Verification items for the finished model (mm, model axes). Face numbers are marked on the shaded views. A direction names the side the tool comes from. Round coordinates to 2 decimals unless told otherwise and drop trailing zeros. Write each loop counter-clockwise with the first axis right and the second up, starting at its lowest first coordinate (ties: lowest second). Pieces come first, ordered by that corner, then holes. Notation, with made-up numbers: M 76.5,68.5 L 116.5,68.5 A33 ccw 116.5,103.5 Z; hole C 39,81 d2. An arc over 180 degrees is marked long. Answer in a Markdown table with one row per item. Add a question column.
1. Go/stop test with flat-tipped pins: pin 1 Ø8 at (x, z) = (-8.5, 4) entering from +Y; pin 2 Ø8 at (y, z) = (13, 12.5) entering from +X; pin 3 Ø5 at (x, z) = (0, -5) entering from -Y; pin 4 Ø5 at (y, z) = (20.5, 10.5) entering from -X. Record where each tip stops, or that it passes through.
2. Material ranges on probe 1 along X at (y, z) = (2.75, -5); probe 2 along X at (y, z) = (6.5, -4); probe 3 along Z at (x, y) = (18.4, 2.75), recorded low to high.
3. Set-up check for the marked faces 5, 6, 7, 8 and 9: record each of +Z, -Z, +X, -X, +Y, -Y from which the full face is reachable in a straight line by a thin tool's end or side.
4. Sectioned sample at A-A on x = 0. Count the separate pieces of the cut face and the enclosed holes in it, plus the area to 3 significant figures.
5. Draft check along Z on the marked faces 1, 2, 3 and 4. Enter one of: pulls with the +Z half, pulls with the -Z half, needs draft (parallel to the pull), parting line crosses it, or undercut.
6. Sectioned sample at B-B on x = -18.4. Record the cut outline in (y, z), plus the area to 3 significant figures.
7. Sectioned sample at D-D on z = -4.5. Record the cut outline in (x, y).
8. Sectioned sample at C-C on y = 20.5. Record the cut outline in (x, z).
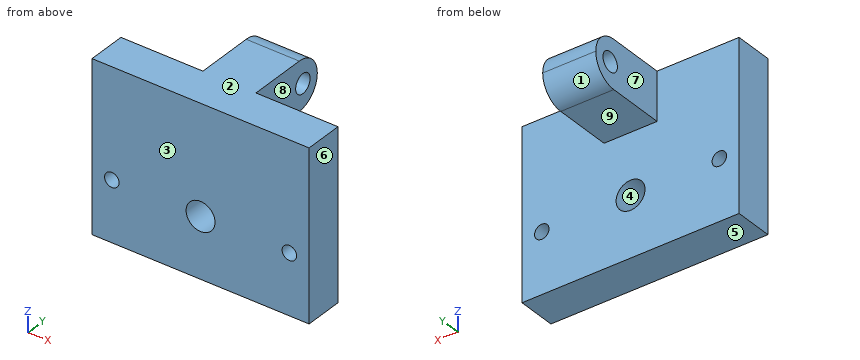
```python
from build123d import *

# Parameters (mm, degrees)
SKETCH2_W           = 45
SKETCH2_H           = 35
SKETCH2_R           = 3
SKETCH2_R_2         = 1.5
BOSS_EXTRUDE1_DEPTH = 5
SKETCH4_R           = 1.5
SKETCH4_R_2         = 3
SKETCH4_W           = 11
SKETCH4_H           = 10
BOSS_EXTRUDE2_DEPTH = 3
SKETCH4_3_W         = 11
SKETCH4_3_H         = 10
BOSS_EXTRUDE3_DEPTH = 20
SKETCH5_R           = 2
CUT_EXTRUDE1_DEPTH  = 20
FILLET1_R           = 5


with BuildPart() as part:
    # Sketch2 → Boss-Extrude1 (new body)
    with BuildSketch(Plane(origin=(0, 0, 0), x_dir=(1, 0, 0), z_dir=(0, 1, 0))):
        Rectangle(SKETCH2_W, SKETCH2_H)
        with Locations(Location((0, 5, 0), (0, 0, 270))):
            Circle(SKETCH2_R, mode=Mode.SUBTRACT)
        with Locations(Location((-18.4, 5, 0), (0, 0, 270))):
            Circle(SKETCH2_R_2, mode=Mode.SUBTRACT)
        with Locations(Location((18.4, 5, 0), (0, 0, 90))):
            Circle(SKETCH2_R_2, mode=Mode.SUBTRACT)
    extrude(amount=BOSS_EXTRUDE1_DEPTH)

    # Sketch4 → Boss-Extrude2 (add)
    # profile 1 of 3: a face of its own
    with BuildSketch(Plane(origin=(0, 5, 0), x_dir=(1, 0, 0), z_dir=(0, 1, 0))):
        Polygon((5.5, -17.5), (15, -17.5), (22.5, -17.5), (22.5, 17.5), (-22.5, 17.5), (-22.5, -17.5), (-15, -17.5), (-5.5, -17.5), (-5.5, -7.5), (5.5, -7.5), align=None)
        with Locations(Location((-18.4, 5, 0), (0, 0, 270))):
            Circle(SKETCH4_R, mode=Mode.SUBTRACT)
        with Locations(Location((0, 5, 0), (0, 0, 270))):
            Circle(SKETCH4_R_2, mode=Mode.SUBTRACT)
        with Locations(Location((18.4, 5, 0), (0, 0, 90))):
            Circle(SKETCH4_R, mode=Mode.SUBTRACT)
    # profile 2 of 3: a face of its own
    with BuildSketch(Plane(origin=(0, 5, 0), x_dir=(1, 0, 0), z_dir=(0, 1, 0))):
        Polygon((5.5, -17.5), (15, -17.5), (22.5, -17.5), (22.5, 17.5), (-22.5, 17.5), (-22.5, -17.5), (-15, -17.5), (-5.5, -17.5), (-5.5, -7.5), (5.5, -7.5), align=None)
        with Locations(Location((-18.4, 5, 0), (0, 0, 270))):
            Circle(SKETCH4_R, mode=Mode.SUBTRACT)
        with Locations(Location((0, 5, 0), (0, 0, 270))):
            Circle(SKETCH4_R_2, mode=Mode.SUBTRACT)
        with Locations(Location((18.4, 5, 0), (0, 0, 90))):
            Circle(SKETCH4_R, mode=Mode.SUBTRACT)
    # profile 3 of 3: a face of its own
    with BuildSketch(Plane(origin=(0, 5, 0), x_dir=(1, 0, 0), z_dir=(0, 1, 0))):
        with Locations((0, -12.5)):
            Rectangle(SKETCH4_W, SKETCH4_H)
    extrude(amount=BOSS_EXTRUDE2_DEPTH)

    # Sketch4<3> → Boss-Extrude3 (add)
    with BuildSketch(Plane(origin=(0, 5, 0), x_dir=(1, 0, 0), z_dir=(0, 1, 0))):
        with Locations((0, -12.5)):
            Rectangle(SKETCH4_3_W, SKETCH4_3_H)
    extrude(amount=BOSS_EXTRUDE3_DEPTH)

    # Sketch5 → Cut-Extrude1 (cut)
    with BuildSketch(Plane(origin=(5.5, 0, 0), x_dir=(0, 0, -1), z_dir=(1, 0, 0))):
        with Locations((-12.5, 21)):
            Circle(SKETCH5_R)
    extrude(amount=-CUT_EXTRUDE1_DEPTH, mode=Mode.SUBTRACT)

    # Fillet1
    fillet1_edges = [part.edges().sort_by_distance(p)[0] for p in [
        (0, 25, 7.5),
        (0, 25, 17.5),
    ]]
    fillet(fillet1_edges, radius=FILLET1_R - 0.0001)  # a hair under: the kernel refuses the full size


solid = part.part
```
Geometry check:
| question | item | result |
|---|---|---|
| 1 | pin 1 | stops at y = 8 |
| 1 | pin 2 | stops at x = 5.5 |
| 1 | pin 3 | passes through |
| 1 | pin 4 | stops at x = -5.5 |
| 2 | probe 1 | x = -22.5 to -19.9, -16.9 to -3, 3 to 16.9, 19.9 to 22.5 |
| 2 | probe 2 | x = -22.5 to -19.52, -17.28 to -2.83, 2.83 to 17.28, 19.52 to 22.5 |
| 2 | probe 3 | z = -17.5 to -6.5, -3.5 to 17.5 |
| 3 | face 5 | -Z, +X, -X, +Y, -Y |
| 3 | face 6 | +Z, -Z, +X, +Y, -Y |
| 3 | face 7 | +Z, -Z, -X, +Y |
| 3 | face 8 | +Z, -Z, +X, +Y |
| 3 | face 9 | -Z, +X, -X, +Y |
| 4 | separate pieces | 2 |
| 4 | enclosed holes | 1 |
| 4 | area | 379 mm2 |
| 5 | face 1 | pulls with the -Z half |
| 5 | face 2 | pulls with the +Z half |
| 5 | face 3 | needs draft |
| 5 | face 4 | undercut |
| 6 | outline | M 0,-17.5 L 8,-17.5 L 8,-6.5 L 0,-6.5 Z; M 0,-3.5 L 8,-3.5 L 8,17.5 L 0,17.5 Z |
| 6 | area | 256 mm2 |
| 7 | outline | M -22.5,0 L -19.81,0 L -19.81,8 L -22.5,8 Z; M -16.99,0 L -2.96,0 L -2.96,8 L -16.99,8 Z; M 2.96,0 L 16.99,0 L 16.99,8 L 2.96,8 Z; M 19.81,0 L 22.5,0 L 22.5,8 L 19.81,8 Z |
| 8 | outline | M -5.5,7.53 L 5.5,7.53 L 5.5,10.56 L -5.5,10.56 Z; M -5.5,14.44 L 5.5,14.44 L 5.5,17.47 L -5.5,17.47 Z |
